Check sheet for the drawn part. Datum: minimum x, y, z corner. Units: mm. Round coordinates to 2 decimals unless told otherwise and drop trailing zeros. Write each loop counter-clockwise with the first axis right and the second up, starting at its lowest first coordinate (ties: lowest second). Pieces come first, ordered by that corner, then holes. Notation, with made-up numbers: M 35,40 L 48,40 A14 ccw 48,45 Z; hole C 65,73 d3. An arc over 180 degrees is marked long. Use a Markdown table: item, result.
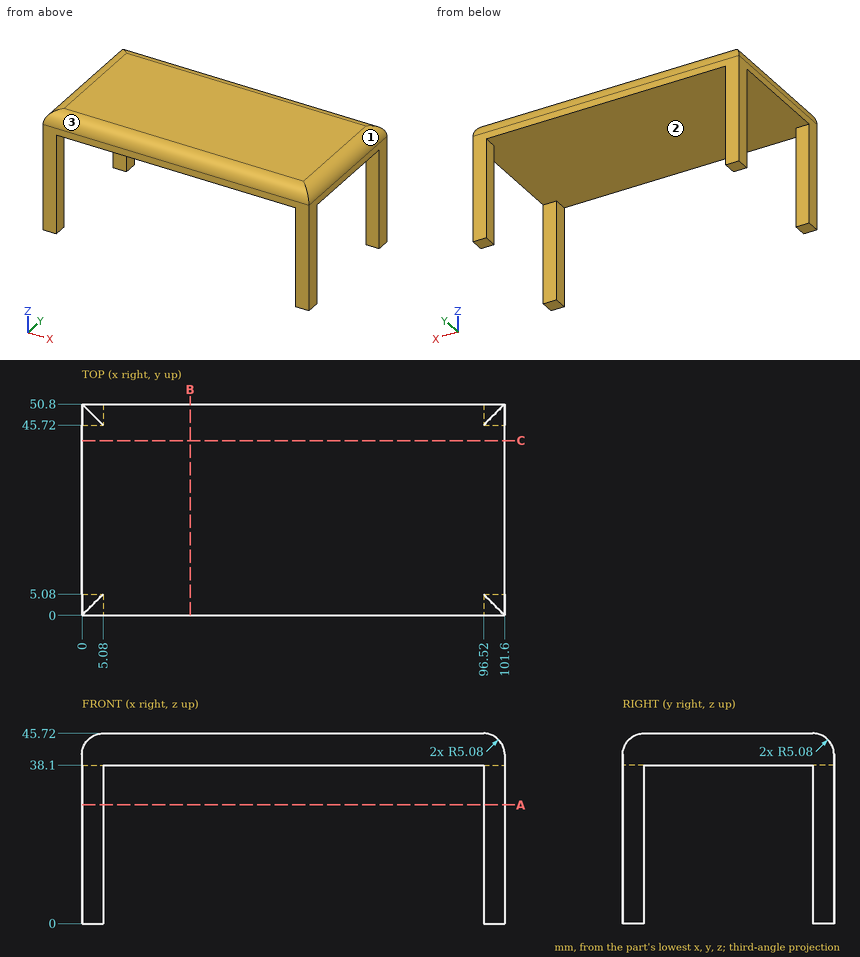
Item 1: Cross-section at B-B, the plane x = 26. Record the cut outline in (y, z), and give its area (3 significant figures).
Outcome:
| item | result |
|---|---|
| outline | M 0,38.1 L 50.8,38.1 L 50.8,40.64 A5.08 ccw 45.72,45.72 L 5.08,45.72 A5.08 ccw 0,40.64 Z |
| area | 376 mm2 |
Item 2: Cross-section at C-C, the plane y = 42. Record the cut outline in (x, z), and give its area (3 significant figures).
Outcome:
| item | result |
|---|---|
| outline | M 0,38.1 L 101.6,38.1 L 101.6,40.64 A5.08 ccw 96.52,45.72 L 5.08,45.72 A5.08 ccw 0,40.64 Z |
| area | 763 mm2 |
Item 3: Go/stop test with flat-tipped pins: pin 1 (6 mm diameter, centred on x = 61, y = 16, fed in from -Z); pin 2 (10 mm diameter, centred on x = 76.5, z = 32.5, fed in from -Y). Record where each tip stops, or that it passes through.
Outcome:
| item | result |
|---|---|
| pin 1 | stops at z = 38.1 |
| pin 2 | passes through |
Item 4: Material ranges on line 1 along X through (y, z) = (46.5, 29); line 2 along Z through (x, y) = (10.5, 37.5); line 3 along X through (y, z) = (12, 41), recorded low to high. Write a range as from..to.
Outcome:
| item | result |
|---|---|
| line 1 | x = 0..5.08, 96.52..101.6 |
| line 2 | z = 38.1..45.72 |
| line 3 | x = 0.01..101.59 |
Item 5: Cross-section at A-A, the plane z = 28.5. Record the cut outline in (x, y), and give its area (3 significant figures).
Outcome:
| item | result |
|---|---|
| outline | M 0,0 L 5.08,0 L 5.08,5.08 L 0,5.08 Z; M 0,45.72 L 5.08,45.72 L 5.08,50.8 L 0,50.8 Z; M 96.52,0 L 101.6,0 L 101.6,5.08 L 96.52,5.08 Z; M 96.52,45.72 L 101.6,45.72 L 101.6,50.8 L 96.52,50.8 Z |
| area | 103 mm2 |
Item 6: Mould release check, pull along X, two halves, no side actions. Record for the marked faces 1, 2 and 3: +X half, -X half, draft (parallel to the pull), parting line (faces both ways), or undercut.
Outcome:
| item | result |
|---|---|
| face 1 | +X half |
| face 2 | undercut |
| face 3 | draft |
